The model under review builds one solid part; all positions refer to its coordinate system, in mm. A direction names the side the tool comes from. Coordinates: 2 decimals unless noted, no trailing zeros. Write each loop counter-clockwise with the first axis right and the second up, starting at its lowest first coordinate (ties: lowest second). Pieces come first, ordered by that corner, then holes. Notation, with made-up numbers: (36, 37.5) - (64, 37.5) arc R18 ccw to (64, 58.5) - close; hole circle Ø11 at (5, 26). An arc over 180 degrees is marked (long way). Put each result on its own line as item: value.
from build123d import *

# Parameters (mm, degrees)
SKETCH_R     = 1.5
PAD_DEPTH    = 4
FILLET_R     = 3
CHAMFER_SIZE = 2


with BuildPart() as part:
    # Sketch → Pad (new body)
    with BuildSketch(Plane.YZ):
        with BuildLine():
            Line((0, 0), (105, 0))
            Line((105, 0), (105, 145))
            ThreePointArc((105, 145), (100.606602, 155.606602), (90, 160))
            Line((0, 160), (90, 160))
            Line((0, 160), (0, 0))
        make_face()
        with Locations((5, 155)):
            Circle(SKETCH_R, mode=Mode.SUBTRACT)
        with Locations((5, 5)):
            Circle(SKETCH_R, mode=Mode.SUBTRACT)
        with Locations((100, 5)):
            Circle(SKETCH_R, mode=Mode.SUBTRACT)
        with Locations((95, 150)):
            Circle(SKETCH_R, mode=Mode.SUBTRACT)
        Polygon((17.30871, 10), (87.69129, 10), (52.5, 70.104262), align=None, mode=Mode.SUBTRACT)
        Polygon((95, 17.30871), (95, 142.69129), (58.293995, 80), align=None, mode=Mode.SUBTRACT)
        Polygon((87.69129, 150), (17.30871, 150), (52.5, 89.895738), align=None, mode=Mode.SUBTRACT)
        Polygon((10, 142.69129), (10, 17.30871), (46.706005, 80), align=None, mode=Mode.SUBTRACT)
    extrude(amount=PAD_DEPTH)

    # Fillet
    fillet_edges = [part.edges().sort_by_distance(p)[0] for p in [
        (2, 52.5, 89.895738),
        (2, 58.293995, 80),
        (2, 52.5, 70.104262),
        (2, 46.706005, 80),
        (2, 17.30871, 150),
        (2, 87.69129, 150),
        (2, 10, 142.69129),
        (2, 95, 142.69129),
        (2, 10, 17.30871),
        (2, 17.30871, 10),
        (2, 95, 17.30871),
        (2, 87.69129, 10),
    ]]
    fillet(fillet_edges, radius=FILLET_R)

    # Chamfer
    chamfer_edges = [part.edges().sort_by_distance(p)[0] for p in [
        (4, 3.5, 155),
        (4, 93.5, 150),
        (4, 98.5, 5),
        (4, 3.5, 5),
    ]]
    chamfer(chamfer_edges, length=CHAMFER_SIZE)


solid = part.part
1. Machinability: for faces 5 (the flat face through (2, 70.3, 39.7)), 6 (the flat face through (2, 0, 81)), which of the approach directions +Z, -Z, +X, -X, +Y, -Y give a long, thin tool a straight path to every point of the face, cutting with its end or side? Answer none if there is none.
Determined:
face 5: +X, -X
face 6: +Z, -Z, +X, -X, -Y
2. Consider section C-C on y = 35.5. State the section outline as (x, z) points.
Determined:
outline: (0, 0) - (4, 0) - (4, 10) - (0, 10) - close; (0, 41.07) - (4, 41.07) - (4, 60.86) - (0, 60.86) - close; (0, 99.14) - (4, 99.14) - (4, 118.93) - (0, 118.93) - close; (0, 150) - (4, 150) - (4, 160) - (0, 160) - close
3. To check wall thickness, follow probe 1 along Z at (x, y) = (0.6, 5); probe 2 along Z at (x, y) = (0.3, 45); probe 3 along Z at (x, y) = (3.1, 32). State the ranges of each line that lie inside material, in increasing order.
Determined:
probe 1: z = 0 to 3.5, 6.5 to 153.5, 156.5 to 160
probe 2: z = 0 to 10, 57.29 to 77.09, 82.91 to 102.71, 150 to 160
probe 3: z = 0 to 10, 35.09 to 54.88, 105.12 to 124.91, 150 to 160
4. The part is to be moulded in two halves that separate along Y. For faces 1 (the flat face through (2, 105, 71)), 2 (the cylindrical face through (0.986, 4.805, 156.487)), 3 (the flat face through (2, 44, 160)), 4 (the cylindrical face through (2.028, 52.456, 67.167)), say which applies: +Y half, -Y half, draft (parallel to the pull), parting line (faces both ways), or undercut.
Determined:
face 1: +Y half
face 2: undercut
face 3: draft
face 4: undercut
5. Consider section B-B on z = 140.5. State the section outline as (x, y) points, plus the area to 3 significant figures.
Determined:
outline: (0, 0) - (4, 0) - (4, 22.87) - (0, 22.87) - close; (0, 82.13) - (4, 82.13) - (4, 105) - (0, 105) - close
area: 183 mm^2
6. Consider section A-A on x = 0.8. Give the number of separate pieces and of enclosed holes in the cut face, plus the area to 3 significant figures.
Determined:
separate pieces: 1
enclosed holes: 8
area: 8,010 mm^2
7. For pin 1 Ø2.5 at (y, z) = (100, 5) entering from +X; pin 2 Ø5 at (y, z) = (95, 150) entering from +X, all flat-tipped, find the tip position at first contact; note any pin that passes through.
Determined:
pin 1: passes through
pin 2: stops at x = 3
